Can you work these out from the model? Positions are in its coordinate system, mm. A direction names the side the tool comes from. Round coordinates to 2 decimals unless told otherwise and drop trailing zeros. Order: outer loops, then holes, each group sorted by start corner. A loop starts at its lowest first (then second) coordinate and runs counter-clockwise, first axis right, second up. Notation, with made-up numbers: (56.25, 44) - (64.25, 44) arc R18 ccw to (64.25, 54) - close; hole circle Ø9 at (77.25, 1). An arc over 180 degrees is marked (long way). Write item = value, one per line.
from build123d import *

# Parameters (mm, degrees)
SKETCH1_W           = 28
SKETCH1_H           = 10.5
SKETCH1_R           = 3.5
SKETCH1_R_2         = 1
SKETCH1_W_2         = 10
SKETCH1_H_2         = 2
BOSS_EXTRUDE1_DEPTH = 5


with BuildPart() as part:
    # Sketch1 → Boss-Extrude1 (new body)
    with BuildSketch(Plane.XY):
        Rectangle(SKETCH1_W, SKETCH1_H)
        Circle(SKETCH1_R, mode=Mode.SUBTRACT)
        with Locations((9.3, 0)):
            Circle(SKETCH1_R_2, mode=Mode.SUBTRACT)
        with Locations((-9.3, 0)):
            Circle(SKETCH1_R_2, mode=Mode.SUBTRACT)
        with Locations((0, 6.25)):
            Rectangle(SKETCH1_W_2, SKETCH1_H_2)
        with Locations((0, -6.25)):
            Rectangle(SKETCH1_W_2, SKETCH1_H_2)
    extrude(amount=BOSS_EXTRUDE1_DEPTH)


solid = part.part
(1) Will these pins go through, and if not, where does the flat tip stop? P1, Ø5.5, axis at x = 0, y = 0, coming from the -Z side; P2, Ø0.6, axis at y = 6.5, z = 2.5, coming from the +X side; P3, Ø1, axis at y = 6.5, z = 1.5, coming from the -X side; P4, Ø2.5, axis at x = -8.5, z = 2, coming from the -Y side.
Computed:
P1 = through
P2 = 5
P3 = -5
P4 = -5.25
(2) On a 3-axis mill with a long thin cutter (end or side, diameter ignored), from which of +Z, -Z, +X, -X, +Y, -Y can I reach the whole of each face in a straight line? I mean faces 1 (the face through (5, 6, 2)), 2 (the face through (-5, 6, 2)), 3 (the face through (9, -5.25, 2)), 4 (the face through (-5, -6, 2)). Say none if no direction works.
Computed:
face_1 = +Z, -Z, +X, +Y
face_2 = +Z, -Z, -X, +Y
face_3 = +Z, -Z, +X, -Y
face_4 = +Z, -Z, -X, -Y
(3) Thinking about a two-plate mould opening in Y: for faces 5 (the face through (-14, 0, 2)), 6 (the face through (0, 7.25, 2)), 7 (the face through (3.233, -1.341, 2.465)), 8 (the face through (-10, -5.25, 2)), which applies, +Y half, -Y half, draft (parallel to the pull), parting line (faces both ways), or undercut?
Computed:
face_5 = draft
face_6 = +Y half
face_7 = undercut
face_8 = -Y half
(4) If we section it at A-A (x = 0): Write out the boundary of the cut face in (y, z), plus the area to 3 significant figures.
Computed:
outline = (-7.25, 0) - (-3.5, 0) - (-3.5, 5) - (-7.25, 5) - close; (3.5, 0) - (7.25, 0) - (7.25, 5) - (3.5, 5) - close
area = 37.5 mm^2
(5) If we section it at D-D (x = -9.3): Write out the boundary of the cut face in (y, z), plus the area to 3 significant figures.
Computed:
outline = (-5.25, 0) - (-1, 0) - (-1, 5) - (-5.25, 5) - close; (1, 0) - (5.25, 0) - (5.25, 5) - (1, 5) - close
area = 42.5 mm^2
(6) If we section it at B-B (y = 0): Write out the boundary of the cut face in (x, z).
Computed:
outline = (-14, 0) - (-10.3, 0) - (-10.3, 5) - (-14, 5) - close; (-8.3, 0) - (-3.5, 0) - (-3.5, 5) - (-8.3, 5) - close; (3.5, 0) - (8.3, 0) - (8.3, 5) - (3.5, 5) - close; (10.3, 0) - (14, 0) - (14, 5) - (10.3, 5) - close
(7) If we section it at C-C (z = 2.35): Write out the boundary of the cut face in (x, y), plus the area to 3 significant figures.
Computed:
outline = (-14, -5.25) - (-5, -5.25) - (-5, -7.25) - (5, -7.25) - (5, -5.25) - (14, -5.25) - (14, 5.25) - (5, 5.25) - (5, 7.25) - (-5, 7.25) - (-5, 5.25) - (-14, 5.25) - close; hole circle Ø2 at (-9.3, 0); hole circle Ø7 at (0, 0); hole circle Ø2 at (9.3, 0)
area = 289 mm^2
(8) If I drill on line 1 (Y direction, x = 9.3, z = 2.9); line 2 (Y direction, x = 0, z = 1.25); line 3 (X direction, y = -0.75, z = 4.3), over which ranges is the centre line in solid material (lowest first)? Write a range as from..to.
Computed:
line_1 = -5.25..-1, 1..5.25
line_2 = -7.25..-3.5, 3.5..7.25
line_3 = -14..-9.96, -8.64..-3.42, 3.42..8.64, 9.96..14
